Study the drawing (mm; zero at the part's minimum x, y, z) and answer. A direction names the side the tool comes from. Give positions to 0.01 mm unless a question says otherwise; leave off trailing zeros. Loops run counter-clockwise (first coordinate to the right, second up) from the corner with the lowest first, then second, coordinate; pieces in that order, holes last. Notation, with made-up numbers: M 28,-32 L 57,-32 A29 ccw 57,-1 Z; hole C 72,71 d2. An arc over 180 degrees is marked long. Return JSON: item names as keys, results as strings.
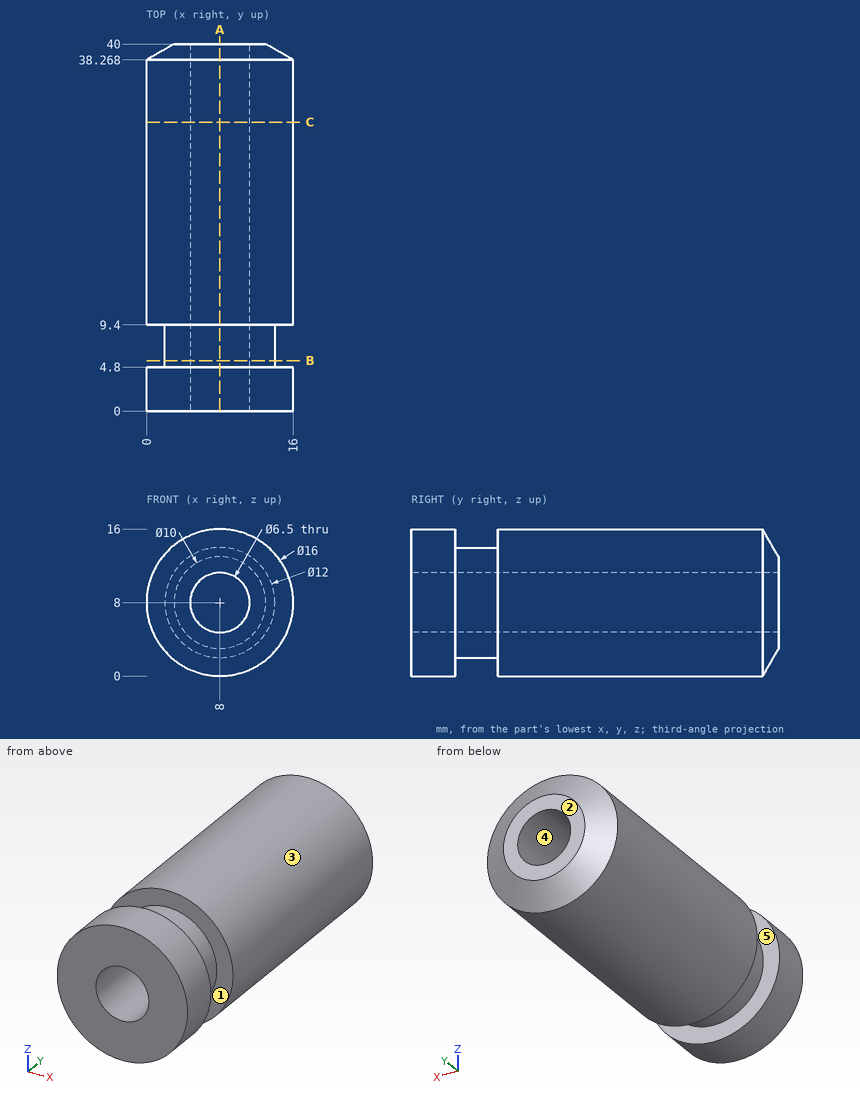
(1) Straight lines are drawn through the part: line 1 along Z through (x, y) = (8, 24); line 2 along X through (y, z) = (36, 7.75); line 3 along Z through (x, y) = (5, 36). For each, find the intervals that lie inside material, in ascending order.
Values follow:
{"line 1": "0 to 4.75, 11.25 to 16", "line 2": "0 to 4.76, 11.24 to 16", "line 3": "0.58 to 6.75, 9.25 to 15.42"}
(2) Given pin 1 (4 mm diameter, centred on x = 8, z = 8, fed in from +Y); pin 2 (2 mm diameter, centred on y = 29.5, z = 4, fed in from -X); pin 3 (1.5 mm diameter, centred on y = 13.5, z = 6.5, fed in from -X); pin 4 (5 mm diameter, centred on y = 30.5, z = 13, fed in from -X), each flat-ended and moving along its own axis, determine where each tip first touches the part or whether it passes through.
Values follow:
{"pin 1": "through", "pin 2": "x = 0.58", "pin 3": "x = 0.04", "pin 4": "x = 0.4"}
(3) The part is cut by section B-B (y = 5.5). Determine the outline of the cut face in (x, z).
Values follow:
{"outline": "C 8,8 d12; hole C 8,8 d6.5"}
(4) The part is cut by section A-A (x = 8). Determine the outline of the cut face in (y, z).
Values follow:
{"outline": "M 0,0 L 4.8,0 L 4.8,2 L 9.4,2 L 9.4,0 L 38.27,0 L 40,3 L 40,4.75 L 0,4.75 Z; M 0,11.25 L 40,11.25 L 40,13 L 38.27,16 L 9.4,16 L 9.4,14 L 4.8,14 L 4.8,16 L 0,16 Z"}
(5) A tool of negligible diameter and unlimited length cuts with its end or side. For the marked faces 1 and 2, from which of +Z, -Z, +X, -X, +Y, -Y can it reach the whole face along a straight path? Write none if from no direction.
Values follow:
{"face 1": "none", "face 2": "+Z, -Z, +X, -X, +Y"}
(6) The part is cut by section C-C (y = 31.5). Determine the outline of the cut face in (x, z), and give its area (3 significant figures).
Values follow:
{"outline": "C 8,8 d16; hole C 8,8 d6.5", "area": "168 mm²"}
(7) Determine the mould class of the marked faces 3, 4 and 5 for opening direction Z: released by +Z, released by -Z, zero draft, split by the parting line, or undercut.
Values follow:
{"face 3": "split by the parting line", "face 4": "undercut", "face 5": "zero draft"}
